Print and shaded views of the part. All mm, measured from the part's lowest x, y and z. Round coordinates to 2 decimals unless told otherwise and drop trailing zeros. Write each loop counter-clockwise with the first axis right and the second up, starting at its lowest first coordinate (ties: lowest second). Pieces come first, ordered by that corner, then holes. Notation, with made-up numbers: (25.5, -10.75) - (68.5, -10.75) arc R20 ccw to (68.5, 17.25) - close; hole circle Ø11 at (-11.75, 85.25). An arc over 180 degrees is marked (long way). Put each result on its own line as item: value. Start each with the question number.
Item 1: Cut at A-A (y = 11). Count the separate pieces of the cut face and the enclosed holes in it.
Item 2: Cut at C-C (x = 3.35). Give the cut face in (y, z), and give its area (3 significant figures).
Item 3: Mould opens along X. For the marked faces 1, 2, 3 and 4 say: released by +X, released by -X, zero draft, split by the parting line, or undercut.
Item 4: Cut at D-D (z = 9.5). Give the cut face in (x, y).
Item 5: Pin check, flat tips, straight feed: pin 1 Ø3.5 at (x, z) = (25.5, 59) entering from +Y; pin 2 Ø1.5 at (x, z) = (12, 35.5) entering from +Y; pin 3 Ø4 at (y, z) = (12, 33.5) entering from +X. Stop position of each tip, or through.
Item 6: Cut at B-B (z = 40). Give the cut face in (x, y).
Item 7: Drill centre lines: line 1 (Z direction, x = 25.62, y = 10.4); line 2 (X direction, y = 10.6, z = 9.5); line 3 (Y direction, x = 61, z = 35). Where is each one in solid material? Low to high. Write a range as from..to.
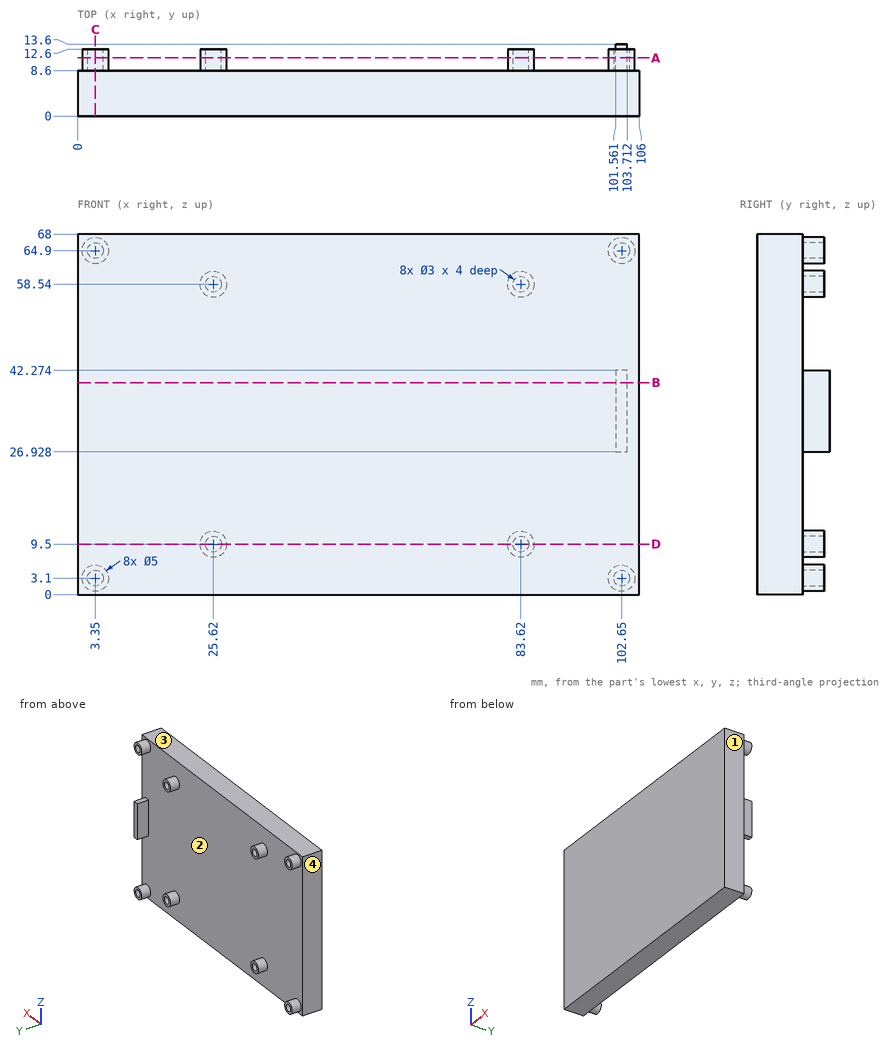
Output values:
1. separate pieces: 9
1. enclosed holes: 8
2. outline: (0, 0) - (8.6, 0) - (8.6, 0.6) - (12.6, 0.6) - (12.6, 1.6) - (8.6, 1.6) - (8.6, 4.6) - (12.6, 4.6) - (12.6, 5.6) - (8.6, 5.6) - (8.6, 62.4) - (12.6, 62.4) - (12.6, 63.4) - (8.6, 63.4) - (8.6, 66.4) - (12.6, 66.4) - (12.6, 67.4) - (8.6, 67.4) - (8.6, 68) - (0, 68) - close
2. area: 601 mm2
3. face 1: released by +X
3. face 2: undercut
3. face 3: zero draft
3. face 4: released by -X
4. outline: (0, 0) - (106, 0) - (106, 8.6) - (86.12, 8.6) - (86.12, 12.6) - (85.12, 12.6) - (85.12, 8.6) - (82.12, 8.6) - (82.12, 12.6) - (81.12, 12.6) - (81.12, 8.6) - (28.12, 8.6) - (28.12, 12.6) - (27.12, 12.6) - (27.12, 8.6) - (24.12, 8.6) - (24.12, 12.6) - (23.12, 12.6) - (23.12, 8.6) - (0, 8.6) - close
5. pin 1: y = 12.6
5. pin 2: y = 8.6
5. pin 3: x = 103.71
6. outline: (0, 0) - (106, 0) - (106, 8.6) - (103.71, 8.6) - (103.71, 13.6) - (101.56, 13.6) - (101.56, 8.6) - (0, 8.6) - close
7. line 1: 7..8, 11..12, 56.04..57.04, 60.04..61.04
7. line 2: 23.12..24.12, 27.12..28.12, 81.12..82.12, 85.12..86.12
7. line 3: 0..8.6
